Work out the finished part from the listing and answer in its coordinate system (mm). A direction names the side the tool comes from. Round coordinates to 2 decimals unless told otherwise and drop trailing zeros. Write each loop counter-clockwise with the first axis right and the second up, starting at its lowest first coordinate (ties: lowest second). Pieces come first, ordered by that corner, then holes. Notation, with made-up numbers: M -22.5,-27 L -7.5,-27 A26 ccw -7.5,-12 Z; hole C 59.5,-16.5 d2. An arc over 180 degrees is marked long. Answer in a Markdown table with one row per item.
```python
from build123d import *

# Parameters (mm, degrees)
F1_DEPTH = 30.48
F3_DEPTH = 60.96
F5_DEPTH = 91.44


with BuildPart() as f1:
    # F0 (on Top) → F1 (new body)
    with BuildSketch(Plane.XY):
        Polygon((-1066.068411, 0), (-1066.068411, -530.347168), (-800.711095, -530.347168), (-800.711095, -271.248341), (-421.450496, -271.248341), (-264.989853, -421.450555), (-264.989853, -1064.816713), (0, -1064.816713), (0, 0), align=None)
    extrude(amount=F1_DEPTH)

    # F2 (on Top) → F3 (join)
    with BuildSketch(Plane.XY):
        Polygon((0, 0), (-685.556054, 0), (0, -684.304416), align=None)
    extrude(amount=F3_DEPTH)

    # F4 (on Top) → F5 (join)
    with BuildSketch(Plane.XY):
        Polygon((0, 0), (-416.443825, 0), (0, -421.450555), align=None)
    extrude(amount=F5_DEPTH)


solid = f1.part
```
1. The part is cut by section C-C (y = -87). Determine the outline of the cut face in (x, z), plus the area to 3 significant figures.
Calculated:
| item | result |
|---|---|
| outline | M -1066.07,0 L 0,0 L 0,91.44 L -330.48,91.44 L -330.48,60.96 L -598.4,60.96 L -598.4,30.48 L -1066.07,30.48 Z |
| area | 60,800 mm² |
2. Determine the mould class of faces 1 (the flat face through (-1066.068, -261, 15)), 2 (the flat face through (-264.99, -739, 15)), 3 (the flat face through (-536, -254, 30.48)) for opening direction X: released by +X, released by -X, zero draft, split by the parting line, or undercut.
Calculated:
| item | result |
|---|---|
| face 1 | released by -X |
| face 2 | undercut |
| face 3 | zero draft |
3. The part is cut by section A-A (x = -354.5). Determine the outline of the cut face in (y, z), plus the area to 3 significant figures.
Calculated:
| item | result |
|---|---|
| outline | M -335.52,0 L 0,0 L 0,91.44 L -62.69,91.44 L -62.69,60.96 L -330.45,60.96 L -330.45,30.48 L -335.52,30.48 Z |
| area | 22,200 mm² |
4. The part is cut by section B-B (y = -860). Determine the outline of the cut face in (x, z), plus the area to 3 significant figures.
Calculated:
| item | result |
|---|---|
| outline | M -264.99,0 L 0,0 L 0,30.48 L -264.99,30.48 Z |
| area | 8,080 mm² |
5. A tool of negligible diameter and unlimited length cuts with its end or side. For faces 4 (the flat face through (-935, -530.347, 15)), 5 (the flat face through (-347.58, -337.36, 45.51)), 6 (the flat face through (-344.315, -345.298, 15.027)), 7 (the flat face through (0, -422, 35)), 8 (the flat face through (-134, -1064.817, 15)), from which of +Z, -Z, +X, -X, +Y, -Y can it reach the whole face along a straight path? Write none if from no direction.
Calculated:
| item | result |
|---|---|
| face 4 | +Z, -Z, -X, -Y |
| face 5 | +Z, -X, -Y |
| face 6 | +Z, -Z, -Y |
| face 7 | +Z, -Z, +X, +Y, -Y |
| face 8 | +Z, -Z, +X, -X, -Y |
6. Given pin 1 (1.5 mm diameter, centred on y = -675, z = 13.5, fed in from -X); pin 2 (3 mm diameter, centred on x = -896.5, y = -207, fed in from -Z); pin 3 (15 mm diameter, centred on x = -989.5, z = 13, fed in from -Y); pin 4 (12 mm diameter, centred on x = -285, z = 71.5, fed in from -Y), each flat-ended and moving along its own axis, determine where each tip first touches the part or whether it passes through.
Calculated:
| item | result |
|---|---|
| pin 1 | stops at x = -264.99 |
| pin 2 | stops at z = 0 |
| pin 3 | stops at y = -530.35 |
| pin 4 | stops at y = -139.1 |
7. Consider line 1 along X through (y, z) = (-491, 5); line 2 along Z through (x, y) = (-75.5, -870); line 3 along Z through (x, y) = (-312, -368.5). Determine where each line is inside the solid, lowest interval first. Write a range as from..to.
Calculated:
| item | result |
|---|---|
| line 1 | x = -1066.07..-800.71, -264.99..0 |
| line 2 | z = 0..30.48 |
| line 3 | z = 0..60.96 |
8. The part is cut by section D-D (x = -715.5). Determine the outline of the cut face in (y, z).
Calculated:
| item | result |
|---|---|
| outline | M -271.25,0 L 0,0 L 0,30.48 L -271.25,30.48 Z |
